Input: part model. Units: mm. Frame: model coordinates. Give positions to 0.01 mm unless a question says otherwise; leave off trailing zeros. Write each loop counter-clockwise with the first axis right and the second up, starting at its lowest first coordinate (ties: lowest second). Pieces come first, ordered by that corner, then holes. Notation, with made-up numbers: (-7, 21.5) -> (27, 21.5) arc R22 cw to (27, 36.5) -> close; hole circle Ø8 at (-20, 24). An arc over 180 degrees is marked (long way). Answer as a JSON object with one key per item and string values. Group by question number.
from build123d import *

# Parameters (mm, degrees)
SKETCH_1_W      = 85
SKETCH_1_H      = 40
EXTRUDE_1_DEPTH = 13.5
FILLET_1_R      = 5


with BuildPart() as part:
    # 草图1 → 凸台-拉伸1 (new, symmetric)
    with BuildSketch(Plane(origin=(0, 0, 0), x_dir=(1, 0, 0), z_dir=(0, 1, 0))):
        Rectangle(SKETCH_1_W, SKETCH_1_H)
    extrude(amount=EXTRUDE_1_DEPTH, both=True)

    # 圆角1
    fillet_1_edges = [part.edges().sort_by_distance(p)[0] for p in [
        (42.5, 13.5, 0),
        (0, 13.5, -20),
        (-42.5, 13.5, 0),
        (0, -13.5, -20),
        (42.5, -13.5, 0),
        (0, -13.5, 20),
        (-42.5, -13.5, 0),
        (0, 13.5, 20),
        (-42.5, 0, -20),
        (42.5, 0, -20),
        (42.5, 0, 20),
        (-42.5, 0, 20),
    ]]
    fillet(fillet_1_edges, radius=FILLET_1_R)


solid = part.part
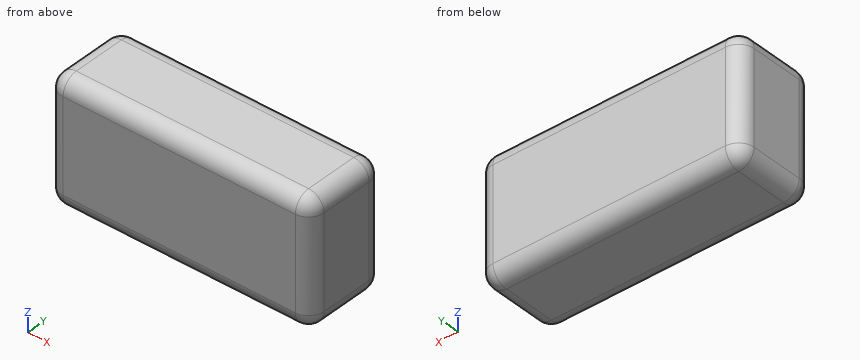
1. Line query: line 1 (Z direction, x = -18, y = 8.75); line 2 (Y direction, x = 38.5, z = -4.5); line 3 (X direction, y = 9.75, z = 4.5). Output: solid intervals per line, ascending.
2. Section B-B (y = 10.5). Return the cut outline in (x, z), plus the area to 3 significant figures.
3. Section A-A (x = -27). Return the cut outline in (y, z).
Working result:
{
 "1": {"line 1": "z = -19.99 to 19.99", "line 2": "y = -13.4 to 13.4", "line 3": "x = -42.34 to 42.34"},
 "2": {"outline": "(-42.08, -15) arc R4.58 ccw to (-37.5, -19.58) -> (37.5, -19.58) arc R4.58 ccw to (42.08, -15) -> (42.08, 15) arc R4.58 ccw to (37.5, 19.58) -> (-37.5, 19.58) arc R4.58 ccw to (-42.08, 15) -> close", "area": "3,280 mm^2"},
 "3": {"outline": "(-13.5, -15) arc R5 ccw to (-8.5, -20) -> (8.5, -20) arc R5 ccw to (13.5, -15) -> (13.5, 15) arc R5 ccw to (8.5, 20) -> (-8.5, 20) arc R5 ccw to (-13.5, 15) -> close"}
}
